Input: dimensioned drawing with shaded views. Units: mm. Origin: part minimum x, y, z. Give positions to 0.01 mm unless a question says otherwise; leave off trailing zeros. Write each loop counter-clockwise with the first axis right and the second up, starting at its lowest first coordinate (ties: lowest second). Pieces come first, ordered by that corner, then holes. Notation, with made-up numbers: (0, -34) - (58, -34) arc R17 cw to (58, -27) - close; hole circle Ø1 at (10.25, -24). An arc over 180 degrees is marked (long way). Answer as CSV lines item,"result".
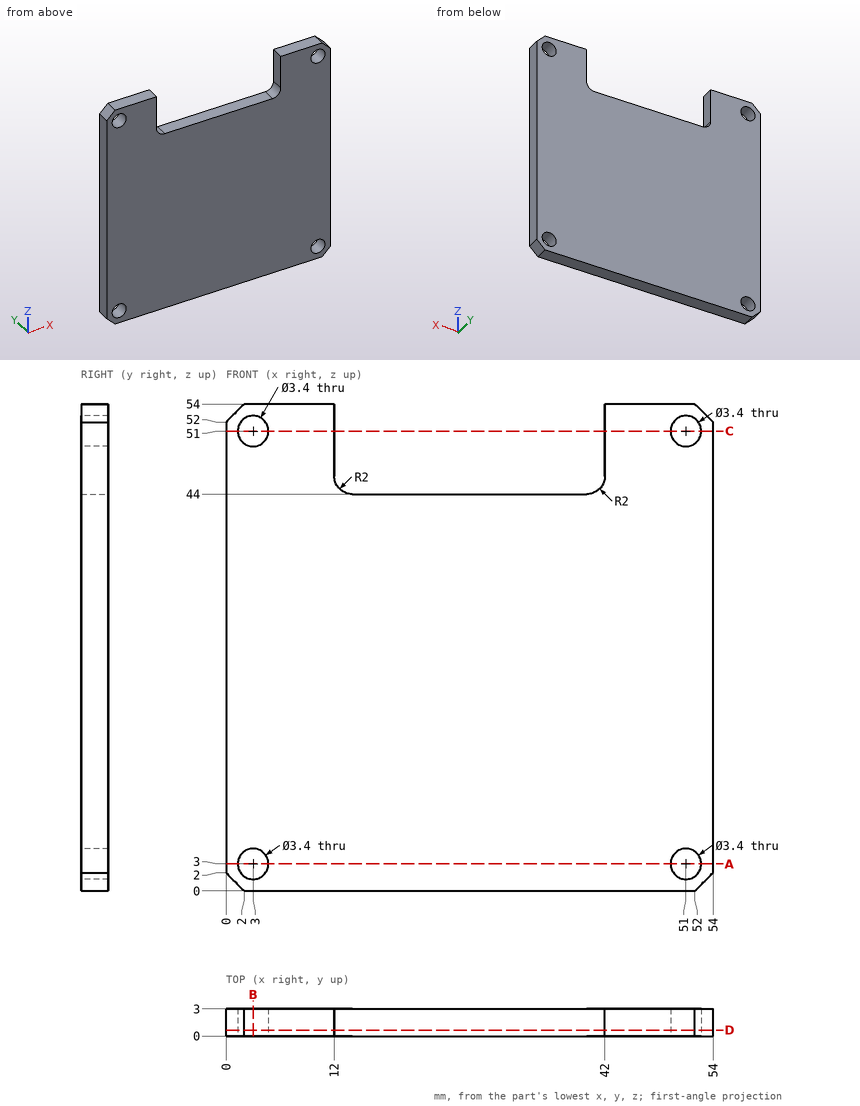
Item 1: Ray query, line 1 (Z direction, x = 3, y = 1.15); line 2 (X direction, y = 1.9, z = 51); line 3 (X direction, y = 0.55, z = 3.5). Return the intervals inside material, ascending. Write a range as from..to.
The answers:
line 1,"0..1.3, 4.7..49.3, 52.7..54"
line 2,"0..1.3, 4.7..12, 42..49.3, 52.7..54"
line 3,"0..1.38, 4.62..49.38, 52.62..54"
Item 2: Cut plane D-D on y = 0.65. Return the cut outline in (x, z), plus the area to 3 significant figures.
The answers:
outline,"(0, 2) - (2, 0) - (52, 0) - (54, 2) - (54, 52) - (52, 54) - (42, 54) - (42, 46) arc R2 cw to (40, 44) - (14, 44) arc R2 cw to (12, 46) - (12, 54) - (2, 54) - (0, 52) - close; hole circle Ø3.4 at (3, 3); hole circle Ø3.4 at (3, 51); hole circle Ø3.4 at (51, 3); hole circle Ø3.4 at (51, 51)"
area,"2,570 mm²"
Item 3: Cut plane C-C on z = 51. Return the cut outline in (x, y).
The answers:
outline,"(0, 0) - (1.3, 0) - (1.3, 3) - (0, 3) - close; (4.7, 0) - (12, 0) - (12, 3) - (4.7, 3) - close; (42, 0) - (49.3, 0) - (49.3, 3) - (42, 3) - close; (52.7, 0) - (54, 0) - (54, 3) - (52.7, 3) - close"
Item 4: Cut plane A-A on z = 3. Return the cut outline in (x, y), plus the area to 3 significant figures.
The answers:
outline,"(0, 0) - (1.3, 0) - (1.3, 3) - (0, 3) - close; (4.7, 0) - (49.3, 0) - (49.3, 3) - (4.7, 3) - close; (52.7, 0) - (54, 0) - (54, 3) - (52.7, 3) - close"
area,"142 mm²"
Item 5: Cut plane B-B on x = 3. Return the cut outline in (y, z), plus the area to 3 significant figures.
The answers:
outline,"(0, 0) - (3, 0) - (3, 1.3) - (0, 1.3) - close; (0, 4.7) - (3, 4.7) - (3, 49.3) - (0, 49.3) - close; (0, 52.7) - (3, 52.7) - (3, 54) - (0, 54) - close"
area,"142 mm²"
Item 6: Contact query for a flat-ended pin moving along its axis: pin 1 (1 mm diameter, centred on x = 18.5, y = 0.5, fed in from +Z). Output: stop coordinate, or through.
The answers:
pin 1,"z = 44"
